```python
from build123d import *

# Parameters (mm, degrees)
F1_DEPTH = 50
F3_DEPTH = 100.001
F4_T     = -2.5


with BuildPart() as f1:
    # F0 (on Front) → F1 (new body)
    with BuildSketch(Plane.XZ):
        Polygon((100, 51.4285714286), (-100, 51.4285714286), (-100, -48.5714285714), (-50, -48.5714285714), (100, 21.4285714286), align=None)
    extrude(amount=F1_DEPTH)

    # F2 (on face) → F3 (cut, through all)
    with BuildSketch(Plane.XY.offset(51.4285714286)):
        Polygon((-121.3779896498, -70.3287050128), (-68.4581929454, -117.7156264903), (-86.6025403784, -50), (-100, -50), (-100, 0), (-122.3772391677, 0), align=None)
        Polygon((-100, -50), (-86.6025403784, -50), (-100, 0), align=None)
    extrude(amount=-F3_DEPTH, mode=Mode.SUBTRACT)

    # F4
    f4_openings = [f1.faces().sort_by_distance(p)[0] for p in [
        (-10.253348, -50, 11.868344),
    ]]
    offset(amount=F4_T, openings=f4_openings)


solid = f1.part
```
Geometry: final body of the model. Coordinates: model frame, mm. A direction names the side the tool comes from. Coordinates: 2 decimals unless noted, no trailing zeros. Order: outer loops, then holes, each group sorted by start corner. A loop starts at its lowest first (then second) coordinate and runs counter-clockwise, first axis right, second up. Notation, with made-up numbers: M -6.75,37.25 L -2.75,37.25 A22 cw -2.75,49.25 Z; hole C 44,7 d9. An arc over 180 degrees is marked long. Answer in a Markdown table with one row per item. Add a question column.
Q1. Section query B-B on z = 43.5. Return the cut outline in (x, y).
Q2. Section query D-D on y = -47. Return the cut outline in (x, z).
Q3. Section query A-A on y = -29. Return the cut outline in (x, z).
Q4. Section query C-C on x = 76.5. Return the cut outline in (y, z).
Q5. Reachability of faces 1 (the flat face through (22.436, -25.918, -12.009)), 2 (the flat face through (-23, -2.5, 13)), 3 (the flat face through (1, -25, 51.429)) from +Z, -Z, +X, -X, +Y, -Y: full face, straight path, thin tool, end or side. Return the list, or none.
Q6. Line query: L1, parallel to Z at x = -79.5, y = -45.5; L2, parallel to Y at x = 26.5, z = 1; L3, parallel to Z at x = -8.5, y = -13.5. Output: solid intervals per line, ascending.
Q7. Mould query, pull axis X, two halves, no side actions, for faces 4 (the flat face through (-70, -25, -48.571)), 5 (the flat face through (-69, -26, -46.071)), 6 (the flat face through (-93.207, -25.35, 2.129)). Classes: released by +X, released by -X, zero draft, split by the parting line, or undercut.
Q8. Contact query for flat-ended pins moving along their axis: P1, Ø10, axis at y = -40, z = -34, coming from the -X side; P2, Ø24, axis at x = -31.5, y = -26, coming from the -Z side; P3, Ø1.5, axis at x = -32.5, y = -22, coming from the -Z side. Output: stop coordinate, or through.
Completed:
| question | item | result |
|---|---|---|
| 1 | outline | M -100,0 L -86.6,-50 L -84.01,-50 L -96.74,-2.5 L 97.5,-2.5 L 97.5,-50 L 100,-50 L 100,0 Z |
| 2 | outline | M -87.41,-48.57 L -50,-48.57 L 100,21.43 L 100,51.43 L -87.41,51.43 Z; hole M -84.82,-46.07 L -50.55,-46.07 L 97.5,23.02 L 97.5,48.93 L -84.82,48.93 Z |
| 3 | outline | M -92.23,-48.57 L -50,-48.57 L 100,21.43 L 100,51.43 L -92.23,51.43 Z; hole M -89.64,-46.07 L -50.55,-46.07 L 97.5,23.02 L 97.5,48.93 L -89.64,48.93 Z |
| 4 | outline | M -50,10.46 L 0,10.46 L 0,51.43 L -50,51.43 L -50,48.93 L -2.5,48.93 L -2.5,13.22 L -50,13.22 Z |
| 5 | face 1 | -Y |
| 5 | face 2 | none |
| 5 | face 3 | +Z, +X, -X, +Y, -Y |
| 6 | L1 | z = -48.57 to -46.07, 48.93 to 51.43 |
| 6 | L2 | y = -2.5 to 0 |
| 6 | L3 | z = -29.2 to -26.45, 48.93 to 51.43 |
| 7 | face 4 | zero draft |
| 7 | face 5 | undercut |
| 7 | face 6 | released by -X |
| 8 | P1 | stops at x = -90.62 |
| 8 | P2 | stops at z = -45.54 |
| 8 | P3 | stops at z = -40.75 |
